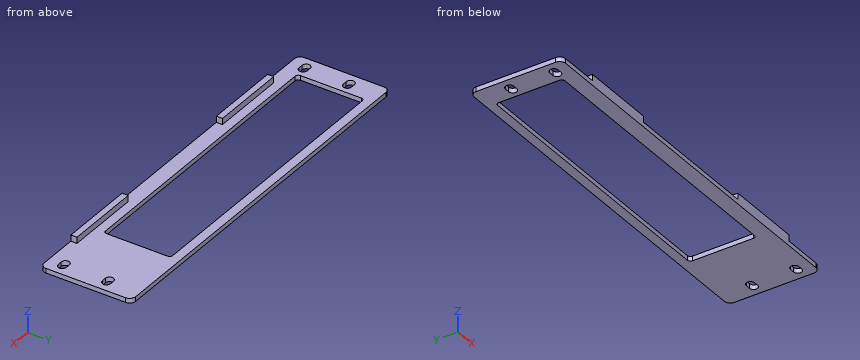
from build123d import *

# Parameters (mm, degrees)
SKETCH1_W           = 252
SKETCH1_H           = 60
BOSS_EXTRUDE1_DEPTH = 3
SKETCH3_W           = 50
SKETCH3_H           = 4
BOSS_EXTRUDE3_DEPTH = 4
SKETCH4_W           = 189
SKETCH4_H           = 44
CUT_EXTRUDE1_DEPTH  = 4
FILLET1_R           = 4
FILLET3_R           = 2


with BuildPart() as part:
    # Sketch1 → Boss-Extrude1 (new body)
    with BuildSketch(Plane.XY):
        with Locations((126, 30)):
            Rectangle(SKETCH1_W, SKETCH1_H)
        with BuildLine():
            Line((245, 36.1), (242, 36.1))
            ThreePointArc((242, 36.1), (239.3, 38.8), (242, 41.5))
            Line((242, 41.5), (245, 41.5))
            ThreePointArc((245, 41.5), (247.7, 38.8), (245, 36.1))
        make_face(mode=Mode.SUBTRACT)
        with BuildLine():
            Line((242, 12.5), (245, 12.5))
            ThreePointArc((245, 12.5), (247.7, 9.8), (245, 7.1))
            Line((245, 7.1), (242, 7.1))
            ThreePointArc((242, 7.1), (239.3, 9.8), (242, 12.5))
        make_face(mode=Mode.SUBTRACT)
        with BuildLine():
            Line((7, 41.5), (10, 41.5))
            ThreePointArc((10, 41.5), (12.7, 38.8), (10, 36.1))
            Line((10, 36.1), (7, 36.1))
            ThreePointArc((7, 36.1), (4.3, 38.8), (7, 41.5))
        make_face(mode=Mode.SUBTRACT)
        with BuildLine():
            Line((7, 12.5), (10, 12.5))
            ThreePointArc((10, 12.5), (12.7, 9.8), (10, 7.1))
            Line((10, 7.1), (7, 7.1))
            ThreePointArc((7, 7.1), (4.3, 9.8), (7, 12.5))
        make_face(mode=Mode.SUBTRACT)
    extrude(amount=BOSS_EXTRUDE1_DEPTH)

    # Sketch3 → Boss-Extrude3 (add)
    with BuildSketch(Plane.XY.offset(3)):
        with Locations((55, 2)):
            Rectangle(SKETCH3_W, SKETCH3_H)
        with Locations((197, 2)):
            Rectangle(SKETCH3_W, SKETCH3_H)
    extrude(amount=BOSS_EXTRUDE3_DEPTH)

    # Sketch4 → Cut-Extrude1 (cut)
    with BuildSketch(Plane.XY.offset(3)):
        with Locations((110.5, 32)):
            Rectangle(SKETCH4_W, SKETCH4_H)
    extrude(amount=-CUT_EXTRUDE1_DEPTH, mode=Mode.SUBTRACT)

    # Fillet1
    fillet1_edges = [part.edges().sort_by_distance(p)[0] for p in [
        (0, 60, 1.5),
        (252, 60, 1.5),
        (252, 0, 1.5),
        (0, 0, 1.5),
    ]]
    fillet(fillet1_edges, radius=FILLET1_R)

    # Fillet3
    fillet3_edges = [part.edges().sort_by_distance(p)[0] for p in [
        (205, 54, 1.5),
        (205, 10, 1.5),
        (16, 10, 1.5),
        (16, 54, 1.5),
    ]]
    fillet(fillet3_edges, radius=FILLET3_R)


solid = part.part
Read the model definition and answer for the solid it produces. Units are mm, in the model's axes. Coordinates: 2 decimals unless noted, no trailing zeros. Loops run counter-clockwise (first coordinate to the right, second up) from the corner with the lowest first, then second, coordinate; pieces in that order, holes last. Notation, with made-up numbers: (60.25, 7.5) -> (108.25, 7.5) arc R34 cw to (108.25, 39.5) -> close; hole circle Ø3 at (7.25, 63). An arc over 180 degrees is marked (long way). Write item = value, one per line. Start each with the question number.
1) The part is cut by section B-B, the plane z = 5.5. Determine the outline of the cut face in (x, y).
2) Given P1, Ø5, axis at x = 223, y = 7.5, coming from the +Z side; P2, Ø2, axis at x = 65.5, z = 6, coming from the +Y side; P3, Ø1.2, axis at y = 1, z = 4.5, coming from the -X side, each flat-ended and moving along its own axis, determine where each tip first touches the part or whether it passes through.
3) The part is cut by section A-A, the plane x = 154. Determine the outline of the cut face in (y, z), plus the area to 3 significant figures.
4) Find the intervals of material crossed by L1, parallel to Y at x = 124.5, z = 2; L2, parallel to X at y = 13, z = 2; L3, parallel to X at y = 40, z = 1, in increasing order. Write a range as from..to.
5) The part is cut by section C-C, the plane y = 38.8. Determine the outline of the cut face in (x, z), plus the area to 3 significant figures.
6) The part is cut by section D-D, the plane x = 65. Determine the outline of the cut face in (y, z).
Result:
q1.outline = (30, 0) -> (80, 0) -> (80, 4) -> (30, 4) -> close; (172, 0) -> (222, 0) -> (222, 4) -> (172, 4) -> close
q2.P1 = 3
q2.P2 = 4
q2.P3 = 30
q3.outline = (0, 0) -> (10, 0) -> (10, 3) -> (0, 3) -> close; (54, 0) -> (60, 0) -> (60, 3) -> (54, 3) -> close
q3.area = 48.0 mm²
q4.L1 = 0..10, 54..60
q4.L2 = 0..16, 205..252
q4.L3 = 0..4.58, 12.42..16, 205..239.58, 247.42..252
q5.outline = (0, 0) -> (4.3, 0) -> (4.3, 3) -> (0, 3) -> close; (12.7, 0) -> (16, 0) -> (16, 3) -> (12.7, 3) -> close; (205, 0) -> (239.3, 0) -> (239.3, 3) -> (205, 3) -> close; (247.7, 0) -> (252, 0) -> (252, 3) -> (247.7, 3) -> close
q5.area = 139 mm²
q6.outline = (0, 0) -> (10, 0) -> (10, 3) -> (4, 3) -> (4, 7) -> (0, 7) -> close; (54, 0) -> (60, 0) -> (60, 3) -> (54, 3) -> close
